Could you check a few things on this drawing? It's one solid part, dimensions in mm from its lowest x, y, z. Give positions to 0.01 mm unless a question says otherwise; leave off trailing zeros. Order: outer loops, then holes, each group sorted by start corner. A loop starts at its lowest first (then second) coordinate and runs counter-clockwise, first axis right, second up. Notation, with made-up numbers: (-38, -3.5) -> (6, -3.5) arc R6 ccw to (6, 4.5) -> close; hole circle Ø3 at (-15, 68.5). An arc over 180 degrees is marked (long way). Write each question's results on one line, items separated by ' | '.
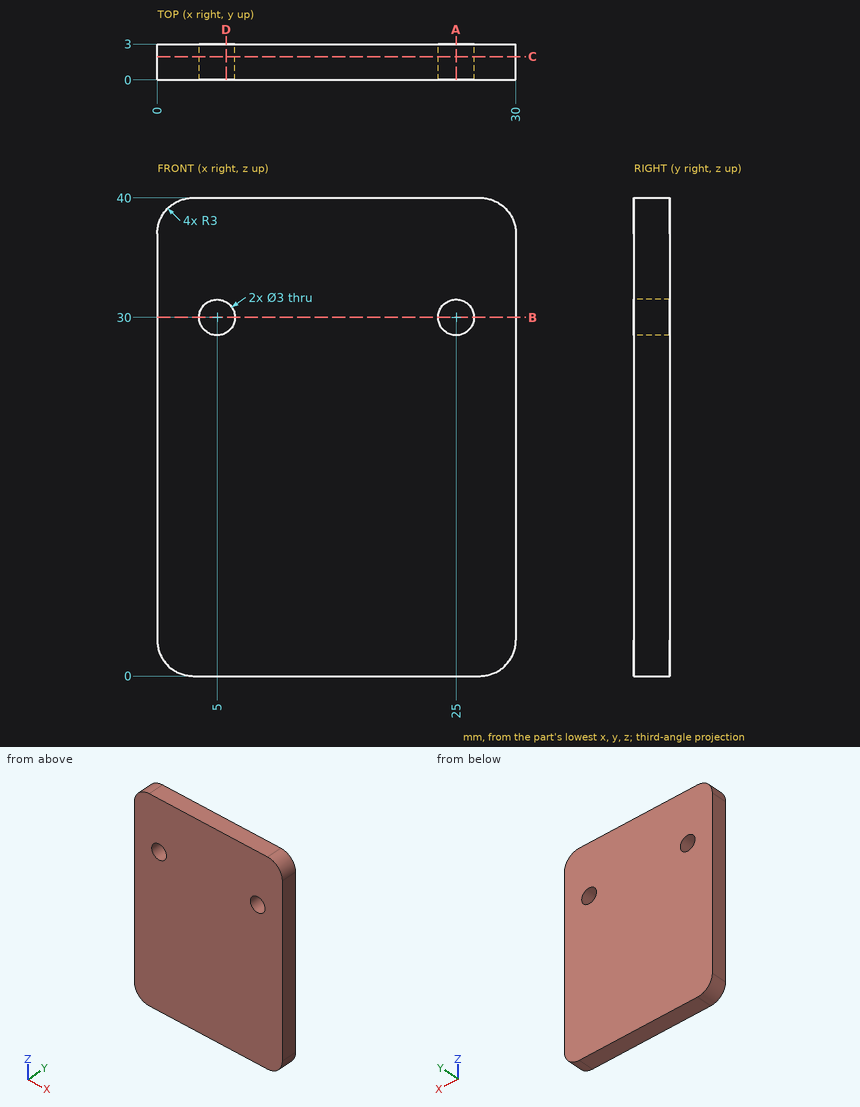
Q1. I need wall thicknesses on line 1 along X through (y, z) = (1.55, 30); line 2 along Z through (x, y) = (25, 2.25); line 3 along X through (y, z) = (0.7, 2). Which ranges of each line are inside material? Lowest first, please.
Here are the results:
line 1: x = 0 to 3.5, 6.5 to 23.5, 26.5 to 30 | line 2: z = 0 to 28.5, 31.5 to 40 | line 3: x = 0.17 to 29.83
Q2. Suppose I cut it at D-D on x = 5.75. Please give me the cut outline in (y, z).
Here are the results:
outline: (0, 0) -> (3, 0) -> (3, 28.7) -> (0, 28.7) -> close; (0, 31.3) -> (3, 31.3) -> (3, 40) -> (0, 40) -> close
Q3. Suppose I cut it at B-B on z = 30. Please give me the cut outline in (x, y).
Here are the results:
outline: (0, 0) -> (3.5, 0) -> (3.5, 3) -> (0, 3) -> close; (6.5, 0) -> (23.5, 0) -> (23.5, 3) -> (6.5, 3) -> close; (26.5, 0) -> (30, 0) -> (30, 3) -> (26.5, 3) -> close
Q4. I'm going to push a flat-ended pin straight in: pin 1 Ø8 at (x, z) = (12.5, 23.5) entering from -Y. Where does the tip first touch, or does it pass through?
Here are the results:
pin 1: stops at y = 0
Q5. Suppose I cut it at A-A on x = 25. Please give me the cut outline in (y, z), and give its area (3 significant figures).
Here are the results:
outline: (0, 0) -> (3, 0) -> (3, 28.5) -> (0, 28.5) -> close; (0, 31.5) -> (3, 31.5) -> (3, 40) -> (0, 40) -> close | area: 111 mm²
Q6. Suppose I cut it at C-C on y = 1.95. Please give me the cut outline in (x, z).
Here are the results:
outline: (0, 3) arc R3 ccw to (3, 0) -> (27, 0) arc R3 ccw to (30, 3) -> (30, 37) arc R3 ccw to (27, 40) -> (3, 40) arc R3 ccw to (0, 37) -> close; hole circle Ø3 at (5, 30); hole circle Ø3 at (25, 30)
